```python
from build123d import *

# Parameters (mm, degrees)
F0_R     = 46.0375
F0_R_2   = 42.8625
F1_DEPTH = 12.7
F0_W     = 8.89
F0_H     = 10.16
F2_DEPTH = 6.35
F3_W     = 10.16
F3_H     = 3.175
F4_DEPTH = 6.6685


with BuildPart() as f1:
    # F0 (on Top) → F1 (new body)
    with BuildSketch(Plane.XY):
        Circle(F0_R)
        Circle(F0_R_2, mode=Mode.SUBTRACT)
    extrude(amount=F1_DEPTH)

    # F0 (on Top) → F2 (join)
    with BuildSketch(Plane.XY):
        Circle(F0_R_2)
        with Locations((-34.925, 0)):
            Rectangle(F0_W, F0_H, mode=Mode.SUBTRACT)
    extrude(amount=F2_DEPTH)

    # F3 (on face) → F4 (cut, through all)
    with BuildSketch(Plane.YZ.offset(-39.37)):
        with Locations((0, 3.175)):
            Rectangle(F3_W, F3_H)
    extrude(amount=-F4_DEPTH, mode=Mode.SUBTRACT)


solid = f1.part
```
Geometry: final body of the model. Coordinates: model frame, mm. A direction names the side the tool comes from. Give positions to 0.01 mm unless a question says otherwise; leave off trailing zeros. Write each loop counter-clockwise with the first axis right and the second up, starting at its lowest first coordinate (ties: lowest second). Pieces come first, ordered by that corner, then holes.
1. Draft query along X for faces 1 (the cylindrical face through (42.53, -17.63, 6.26)), 2 (the flat face through (-37, 5.08, 3)), 3 (the flat face through (-30.48, 0, 3)), 4 (the flat face through (-43, 0, 1.588)). Return one class per face: released by +X, released by -X, zero draft, split by the parting line, or undercut.
2. Section query D-D, the plane y = -25.5. Return loops of the section in (x, z).
3. Pin query (flat end, axial travel): P1, Ø7, axis at x = -36.5, z = 3.5, coming from the -Y side; P2, Ø5, axis at y = -34, z = 10.5, coming from the -X side; P3, Ø7.5, axis at x = -43.5, y = -0.5, coming from the -Z side; P4, Ø10, axis at x = -29, y = 5.5, coming from the +Z side. Return the tip coordinate at first contact, or that it passes through.
4. Section query B-B, the plane z = 8.75. Return loops of the section in (x, y) (1 decimal).
5. Section query A-A, the plane y = 0. Return loops of the section in (x, z), then the cut area to 3 significant figures.
6. Reachability of faces 5 (the flat face through (-37, -5.08, 3)), 6 (the flat face through (-1, 1, 6.35)), 7 (the flat face through (-43, 0, 4.762)) from +Z, -Z, +X, -X, +Y, -Y: full face, straight path, thin tool, end or side. Return the list, or none.
7. Section query C-C, the plane x = 0. Return loops of the section in (y, z).
8. Line query: probe 1 along X at (y, z) = (1, 1.25); probe 2 along Y at (x, z) = (0, 10); probe 3 along Z at (x, y) = (-35.5, -12.5). Output: solid intervals per line, ascending.
Computed:
1. face 1: split by the parting line
1. face 2: undercut
1. face 3: undercut
1. face 4: zero draft
2. outline: (-38.33, 0) - (38.33, 0) - (38.33, 12.7) - (34.45, 12.7) - (34.45, 6.35) - (-34.45, 6.35) - (-34.45, 12.7) - (-38.33, 12.7) - close
3. P1: stops at y = -32.1
3. P2: stops at x = -33.57
3. P3: stops at z = 0
3. P4: stops at z = 6.35
4. outline: circle Ø92.1 at (0, 0); hole circle Ø85.7 at (0, 0)
5. outline: (-46.04, 0) - (-39.37, 0) - (-39.37, 1.59) - (-46.04, 1.59) - close; (-46.04, 4.76) - (-39.37, 4.76) - (-39.37, 6.35) - (-42.86, 6.35) - (-42.86, 12.7) - (-46.04, 12.7) - close; (-30.48, 0) - (46.04, 0) - (46.04, 12.7) - (42.86, 12.7) - (42.86, 6.35) - (-30.48, 6.35) - close
5. area: 547 mm2
6. face 5: none
6. face 6: +Z
6. face 7: -X
7. outline: (-46.04, 0) - (46.04, 0) - (46.04, 12.7) - (42.86, 12.7) - (42.86, 6.35) - (-42.86, 6.35) - (-42.86, 12.7) - (-46.04, 12.7) - close
8. probe 1: x = -46.03 to -39.37, -30.48 to 46.03
8. probe 2: y = -46.04 to -42.86, 42.86 to 46.04
8. probe 3: z = 0 to 6.35
